Autodesk Inventor part; units mm, degrees
ref_plane "YZ Plane" through (0, 0, 0) normal (1, 0, 0) x (0, 1, 0)
ref_plane "XZ Plane" through (0, 0, 0) normal (0, 1, 0) x (-1, 0, 0)
ref_plane "XY Plane" through (0, 0, 0) normal (0, 0, 1) x (1, 0, 0)
sketch "Sketch1" plane through (0, 0, 0) normal (0, 0, 1) x (1, 0, 0)
  line L0 (20, 50) -> (20, -50)
  line L1 (10, -60) -> (-10, -60)
  line L2 (-20, -50) -> (-20, 50)
  arc A0 (10, -60) -> (20, -50) centre (10, -50) ccw
  arc A1 (-20, -50) -> (-10, -60) centre (-10, -50) ccw
  line L3 (-20, 80) -> (-20, 50)
  line L4 (20, 80) -> (20, 50)
  line L5 (-20, 80) -> (-100, 80) construction
  arc A2 (-20, 80) -> (-100, 160) centre (-100, 80) ccw
  arc A3 (20, 80) -> (-100, 200) centre (-100, 80) ccw
  line L6 (-100, 160) -> (-123.094, 200)
  line L7 (-100, 160) -> (-53.812, 160) construction
  line L8 (-123.094, 200) -> (-100, 200)
  point P0 (0, 0)
  point P1 (20, 0)
  point P2 (0, 80)
  dimension "d1" = 40
  dimension "d11" = 80
  dimension "d12" = 140
  dimension "d19" = 120
extrude "Extrusion1" add sketch "Sketch1" along normal blind 5
sketch "Sketch3" plane through (0, 0, 5) normal (0, 0, 1) x (1, 0, 0)
  circle A0 centre (0, -50) radius 5
  line L0 (-10, -60) -> (10, -60)
  circle A1 centre (0, 30) radius 5
  point P0 (0, 0)
  dimension "d13" = 10
  dimension "d14" = 10
  dimension "d15" = 10
  dimension "d16" = 80
extrude "Extrusion3" cut sketch "Sketch3" against normal up to surface (5 mm away)
equation "\"d17\" = d13"
properties part number "garrita"
Source: CAD feature listing. Evaluate the final solid. Frame: model axes, mm. Give positions to 0.01 mm unless a question says otherwise; leave off trailing zeros. Loops run counter-clockwise (first coordinate to the right, second up) from the corner with the lowest first, then second, coordinate; pieces in that order, holes last. Notation, with made-up numbers: (3.5, -10) -> (47.5, -10) arc R10 cw to (47.5, -5) -> close; hole circle Ø1 at (85, 46). An arc over 180 degrees is marked (long way). Put each result on its own line as item: value. Start each with the question number.
1) Cut plane A-A (y = 30). Return loops of the section in (x, z).
2) Cut plane B-B (x = 0). Return loops of the section in (y, z).
3) Draft query along X for faces 1 (the face through (-1.08, 25.12, 2.54)), 2 (the face through (-20, 14, 2)), 3 (the face through (20, 16, 2)). Return one class per face: released by +X, released by -X, zero draft, split by the parting line, or undercut.
4) Contact query for flat-ended pins moving along their axis: P1, Ø3, axis at y = 6.5, z = 4.5, coming from the -X side; P2, Ø1.5, axis at x = -45, z = 2.5, coming from the +Y side. Output: stop coordinate, or through.
5) Cut plane C-C (y = -24). Return loops of the section in (x, z), then the cut area to 3 significant figures.
6) Material intervals for probe 1 along Y at (x, z) = (0, 2.1); probe 2 along X at (y, z) = (5, 1.6); probe 3 along Y at (x, z) = (-106.5, 1.9), sorted ascending.
7) Cut plane D-D (x = -36). Return loops of the section in (y, z).
Results are:
1. outline: (-20, 0) -> (-5, 0) -> (-5, 5) -> (-20, 5) -> close; (5, 0) -> (20, 0) -> (20, 5) -> (5, 5) -> close
2. outline: (-60, 0) -> (-55, 0) -> (-55, 5) -> (-60, 5) -> close; (-45, 0) -> (25, 0) -> (25, 5) -> (-45, 5) -> close; (35, 0) -> (146.33, 0) -> (146.33, 5) -> (35, 5) -> close
3. face 1: undercut
3. face 2: released by -X
3. face 3: released by +X
4. P1: stops at x = -20
4. P2: stops at y = 187.04
5. outline: (-20, 0) -> (20, 0) -> (20, 5) -> (-20, 5) -> close
5. area: 200 mm2
6. probe 1: y = -60 to -55, -45 to 25, 35 to 146.33
6. probe 2: x = -20 to 20
6. probe 3: y = 171.26 to 200
7. outline: (128, 0) -> (181.51, 0) -> (181.51, 5) -> (128, 5) -> close
